Study the drawing (mm; zero at the part's minimum x, y, z) and answer. A direction names the side the tool comes from. Round coordinates to 2 decimals unless told otherwise and drop trailing zeros. Order: outer loops, then holes, each group sorted by start corner. A loop starts at its lowest first (then second) coordinate and runs counter-clockwise, first axis right, second up. Notation, with made-up numbers: M 60,-13.75 L 104,-13.75 A20 ccw 104,-4.75 Z; hole C -36,38.5 d11. An arc over 180 degrees is marked long. Put each result on its own line as item: value. Start each with the question number.
1. Which of the six approach directions +Z, -Z, +X, -X, +Y, -Y give full straight-line access (tool end or side, diameter ignored) to the marked faces 4 and 5?
2. The part is cut by section A-A (z = 3). Give the vertices of the cut face in (x, y), then the cut area to 3 significant figures.
3. The part is cut by section B-B (y = 47.5). Give the vertices of the cut face in (x, z), then the cut area to 3 significant figures.
4. The mould has two halves that part along Y. Classify the marked faces 1, 2 and 3: +Y half, -Y half, draft (parallel to the pull), parting line (faces both ways), or undercut.
5. Consider line 1 (X direction, y = 18, z = 2.25); line 2 (Y direction, x = 38.5, z = 4.25). Determine where each line is inside the solid, lowest interval first.
6. Each of these flat-tipped pins is pushed along its axis until it touches: pin 1 Ø3 at (x, z) = (18, 5.5) entering from -Y; pin 2 Ø8 at (x, y) = (38.5, 12.5) entering from +Z. Where does it stop, or does it pass through?
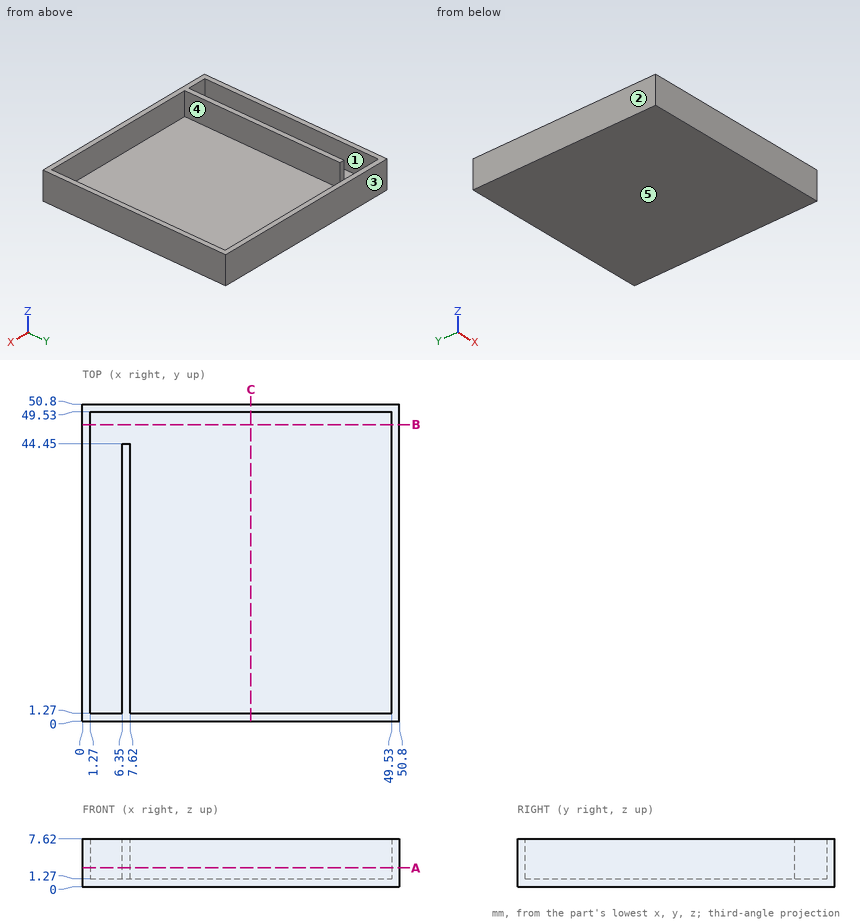
Resolved:
1. face 4: +Z
1. face 5: -Z, +X, -X, +Y, -Y
2. outline: M 0,0 L 50.8,0 L 50.8,50.8 L 0,50.8 Z; hole M 1.27,1.27 L 6.35,1.27 L 6.35,44.45 L 7.62,44.45 L 7.62,1.27 L 49.53,1.27 L 49.53,49.53 L 1.27,49.53 Z
2. area: 306 mm2
3. outline: M 0,0 L 50.8,0 L 50.8,7.62 L 49.53,7.62 L 49.53,1.27 L 1.27,1.27 L 1.27,7.62 L 0,7.62 Z
3. area: 80.6 mm2
4. face 1: undercut
4. face 2: draft
4. face 3: +Y half
5. line 1: 0 to 1.27, 6.35 to 7.62, 49.53 to 50.8
5. line 2: 0 to 1.27, 49.53 to 50.8
6. pin 1: y = 0
6. pin 2: z = 1.27
